Check sheet for the drawn part. Datum: minimum x, y, z corner. Units: mm. A direction names the side the tool comes from. Give positions to 0.01 mm unless a question says otherwise; leave off trailing zeros. Write each loop counter-clockwise with the first axis right and the second up, starting at its lowest first coordinate (ties: lowest second). Pieces come first, ordered by that corner, then holes. Notation, with made-up numbers: (-22, 7.5) - (-4, 7.5) arc R11 cw to (-4, 22.5) - close; hole circle Ø3 at (-37.5, 20.5). An arc over 180 degrees is marked (long way). Answer as a JSON object with one key per item and string values. Group by question number.
Item 1: Go/stop test with flat-tipped pins: pin 1 (5 mm diameter, centred on y = 8.5, z = 14, fed in from +X); pin 2 (3 mm diameter, centred on x = 10, y = 19, fed in from -Z); pin 3 (9.5 mm diameter, centred on x = 11, y = 17, fed in from -Z). Record where each tip stops, or that it passes through.
Item 2: Sectioned sample at B-B, the plane z = 6. Record the boundary of the cut face in (x, y), and give its area (3 significant figures).
Item 3: Scan lines: line 1 along Y through (x, z) = (10, 18.55); line 2 along X through (y, z) = (0.7, 6); line 3 along Z through (x, y) = (10, 1.45). Record each from-to range of solid material in increasing order. Write a range as [from, to].
Item 4: Tool access check on the marked faces 4 and 5. Record the directions out of +Z, -Z, +X, -X, +Y, -Y that give a thin tool (end or side, any length) a straight path to the whole face; none if there is none.
Item 5: Draft check along X on the marked faces 1, 2 and 3. Enter one of: +X half, -X half, draft (parallel to the pull), parting line (faces both ways), or undercut.
Item 6: Sectioned sample at D-D, the plane x = 3.25. Record the boundary of the cut face in (y, z).
Item 7: Sectioned sample at C-C, the plane x = 10. Record the boundary of the cut face in (y, z), and give its area (3 significant figures).
Item 8: Sectioned sample at A-A, the plane y = 12. Record the boundary of the cut face in (x, z).
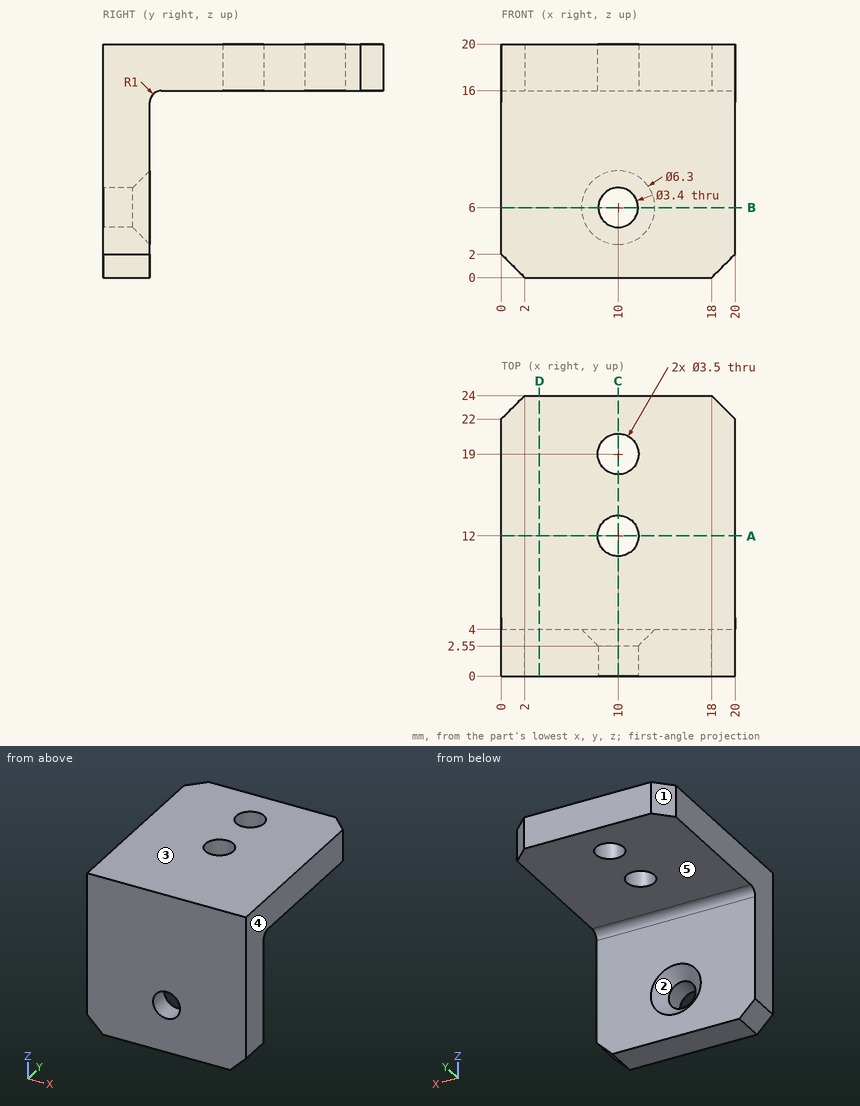
Geometry check:
{
 "1": {"pin 1": "x = 20", "pin 2": "through", "pin 3": "z = 16"},
 "2": {"outline": "(0, 0) - (8.3, 0) - (8.3, 2.55) - (6.85, 4) - (0, 4) - close; (11.7, 0) - (20, 0) - (20, 4) - (13.15, 4) - (11.7, 2.55) - close", "area": "64.3 mm^2"},
 "3": {"line 1": "[0, 10.25], [13.75, 17.25], [20.75, 24]", "line 2": "[0, 8.3], [11.7, 20]", "line 3": "[0, 4.3], [7.7, 20]"},
 "4": {"face 4": "+Z, -Z, +X, +Y, -Y", "face 5": "-Z, +X, -X, +Y"},
 "5": {"face 1": "-X half", "face 2": "undercut", "face 3": "draft"},
 "6": {"outline": "(0, 0) - (4, 0) - (4, 15) arc R1 cw to (5, 16) - (24, 16) - (24, 20) - (0, 20) - close"},
 "7": {"outline": "(0, 0) - (4, 0) - (4, 2.85) - (2.55, 4.3) - (0, 4.3) - close; (0, 7.7) - (2.55, 7.7) - (4, 9.15) - (4, 15) arc R1 cw to (5, 16) - (10.25, 16) - (10.25, 20) - (0, 20) - close; (13.75, 16) - (17.25, 16) - (17.25, 20) - (13.75, 20) - close; (20.75, 16) - (24, 16) - (24, 20) - (20.75, 20) - close", "area": "117 mm^2"},
 "8": {"outline": "(0, 16) - (8.25, 16) - (8.25, 20) - (0, 20) - close; (11.75, 16) - (20, 16) - (20, 20) - (11.75, 20) - close"}
}
